Verification items for the finished model (mm, model axes). Face numbers are marked on the shaded views. Give positions to 0.01 mm unless a question says otherwise; leave off trailing zeros. Loops run counter-clockwise (first coordinate to the right, second up) from the corner with the lowest first, then second, coordinate; pieces in that order, holes last. Notation, with made-up numbers: M 60,47 L 70,47 A4 ccw 70,54 Z; hole C -25.75,-14.75 d2. An arc over 180 degrees is marked long. Put each result on its own line as item: value. Start each with the question number.
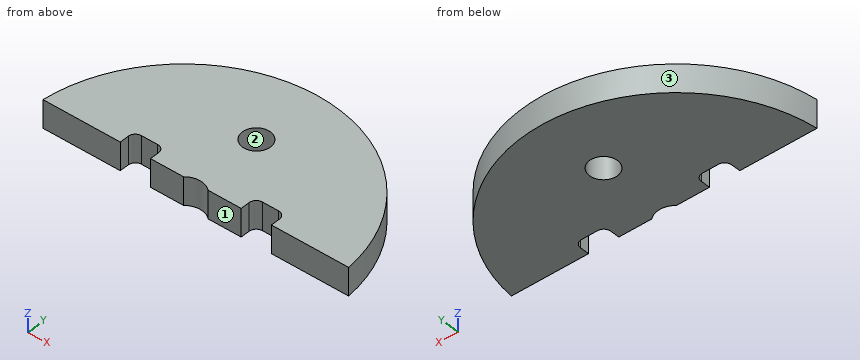
from build123d import *

# Parameters (mm, degrees)
MODEL_R                 = 1.5
SALIENTE_EXTRUIR1_DEPTH = 3


with BuildPart() as part:
    # Model → Saliente-Extruir1 (new body)
    with BuildSketch(Plane.XY):
        with BuildLine():
            Line((223.122807913, 245.202019993), (221.372807913, 245.202019993))
            ThreePointArc((221.372807913, 245.202019993), (220.842477828, 244.982350079), (220.622807913, 244.452019993))
            Line((220.622807913, 244.452019993), (220.622807913, 243.452019993))
            Line((220.622807913, 243.452019993), (217.070683569, 243.452019993))
            ThreePointArc((217.070683569, 243.452019993), (215.747807914, 243.952019993), (214.424932258, 243.452019993))
            Line((214.424932258, 243.452019993), (210.872807913, 243.452019993))
            Line((210.872807913, 243.452019993), (210.872807913, 244.452019993))
            ThreePointArc((210.872807913, 244.452019993), (210.653137999, 244.982350079), (210.122807913, 245.202019993))
            Line((210.122807913, 245.202019993), (208.372807913, 245.202019993))
            ThreePointArc((208.372807913, 245.202019993), (207.842477828, 244.982350079), (207.622807913, 244.452019993))
            Line((207.622807913, 244.452019993), (207.622807913, 243.452019993))
            Line((207.622807913, 243.452019993), (199.316131188, 243.452019993))
            ThreePointArc((199.316131188, 243.452019993), (215.747807914, 258.452019993), (232.179484639, 243.452019993))
            Line((232.179484639, 243.452019993), (223.872807913, 243.452019993))
            Line((223.872807913, 243.452019993), (223.872807913, 244.452019993))
            ThreePointArc((223.872807913, 244.452019993), (223.653137999, 244.982350079), (223.122807913, 245.202019993))
        make_face()
        with Locations((215.747807914, 250.952019993)):
            Circle(MODEL_R, mode=Mode.SUBTRACT)
    extrude(amount=SALIENTE_EXTRUIR1_DEPTH)


solid = part.part
Q1. Go/stop test with flat-tipped pins: pin 1 (6 mm diameter, centred on x = 223, y = 255.5, fed in from -Z); pin 2 (1.8 mm diameter, centred on x = 215.75, y = 250.95, fed in from +Z); pin 3 (0.9 mm diameter, centred on x = 222, z = 1, fed in from -Y); pin 4 (1 mm diameter, centred on x = 220.5, z = 1, fed in from +Y). Record where each tip stops, or that it passes through.
Q2. Cross-section at A-A, the plane z = 1.7. Record the boundary of the cut face in (x, y), then the cut area to 3 significant figures.
Q3. Cross-section at C-C, the plane x = 225.5. Record the boundary of the cut face in (y, z).
Q4. Release check for a two-part mould opening along X. For the marked faces 1, 2 and 3 record: pulls with the +X half, pulls with the -X half, needs draft (parallel to the pull), parting line crosses it, or undercut.
Q5. Scan lines: L1, parallel to X at y = 249.75, z = 2.35; L2, parallel to X at y = 250, z = 2.35; L3, parallel to Y at x = 219.5, z = 2.9. Record each from-to range of solid material in increasing order.
Q6. Cross-section at B-B, the plane y = 254.5. Record the boundary of the cut face in (x, z), then the cut area to 3 significant figures.
Ans:
1. pin 1: stops at z = 0
1. pin 2: passes through
1. pin 3: stops at y = 245.2
1. pin 4: stops at y = 257.89
2. outline: M 199.32,243.45 L 207.62,243.45 L 207.62,244.45 A0.75 cw 208.37,245.2 L 210.12,245.2 A0.75 cw 210.87,244.45 L 210.87,243.45 L 214.42,243.45 A2 cw 217.07,243.45 L 220.62,243.45 L 220.62,244.45 A0.75 cw 221.37,245.2 L 223.12,245.2 A0.75 cw 223.87,244.45 L 223.87,243.45 L 232.18,243.45 A16.5 ccw Z; hole C 215.75,250.95 d3
2. area: 359 mm^2
3. outline: M 243.45,0 L 255.26,0 L 255.26,3 L 243.45,3 Z
4. face 1: needs draft
4. face 2: undercut
4. face 3: parting line crosses it
5. L1: x = 201.21 to 214.85, 216.65 to 230.29
5. L2: x = 201.34 to 214.59, 216.91 to 230.15
5. L3: y = 243.45 to 258.02
6. outline: M 205.03,0 L 226.46,0 L 226.46,3 L 205.03,3 Z
6. area: 64.3 mm^2
